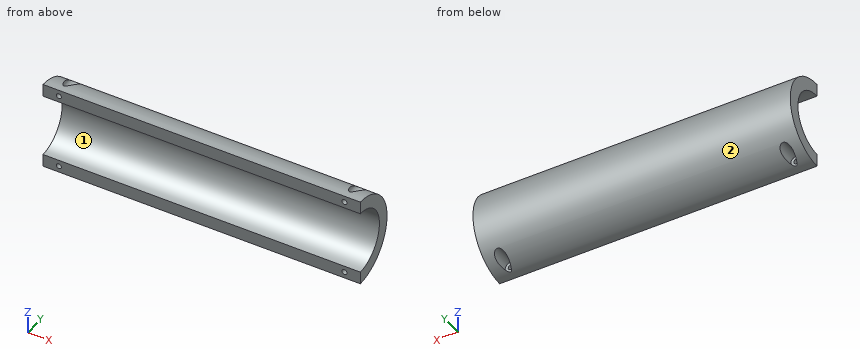
from build123d import *

# Parameters (mm, degrees)
AUFSATZ_LINEAR_AUSTRAGEN1_DEPTH = 200
SKIZZE2_R                       = 1.6
SCHNITT_LINEAR_AUSTRAGEN1_DEPTH = 204.882318998
SCHNITT_LINEAR_START            = -5
SKIZZE3_R                       = 3.5
SCHNITT_LINEAR_AUSTRAGEN2_DEPTH = 199.882319124


with BuildPart() as part:
    # Skizze1 → Aufsatz-Linear austragen1 (new body)
    with BuildSketch(Plane(origin=(0, 0, 0), x_dir=(0, 0, -1), z_dir=(1, 0, 0))):
        with BuildLine():
            Line((-28, 0), (-20, 0))
            ThreePointArc((-20, 0), (0, 20), (20, 0))
            Line((20, 0), (28, 0))
            ThreePointArc((28, 0), (0, 28), (-28, 0))
        make_face()
    extrude(amount=AUFSATZ_LINEAR_AUSTRAGEN1_DEPTH)

    # Skizze2 → Schnitt-Linear austragen1 (cut, through all)
    with BuildSketch(Plane.XZ):
        with Locations(Location((10, 24, 0), (0, 0, 270))):
            Circle(SKIZZE2_R)
        with Locations(Location((190, 24, 0), (0, 0, 270))):
            Circle(SKIZZE2_R)
        with Locations(Location((190, -24, 0), (0, 0, 270))):
            Circle(SKIZZE2_R)
        with Locations(Location((10, -24, 0), (0, 0, 270))):
            Circle(SKIZZE2_R)
    extrude(amount=-SCHNITT_LINEAR_AUSTRAGEN1_DEPTH, mode=Mode.SUBTRACT)

    # Skizze3 → Schnitt-Linear austragen2 (cut, through all)
    with BuildSketch(Plane.XZ.offset(SCHNITT_LINEAR_START)):
        with Locations(Location((10, 24, 0), (0, 0, 270))):
            Circle(SKIZZE3_R)
        with Locations(Location((190, 24, 0), (0, 0, 270))):
            Circle(SKIZZE3_R)
        with Locations(Location((190, -24, 0), (0, 0, 270))):
            Circle(SKIZZE3_R)
        with Locations(Location((10, -24, 0), (0, 0, 270))):
            Circle(SKIZZE3_R)
    extrude(amount=-SCHNITT_LINEAR_AUSTRAGEN2_DEPTH, mode=Mode.SUBTRACT)


solid = part.part
CAD build for the part. Positions are in the model's coordinates, mm. Face numbers are marked on the shaded views. Round coordinates to 2 decimals unless told otherwise and drop trailing zeros. Loops run counter-clockwise (first coordinate to the right, second up) from the corner with the lowest first, then second, coordinate; pieces in that order, holes last. Notation, with made-up numbers: M 72.5,-0.5 L 90.5,-0.5 A16 ccw 90.5,6.5 Z; hole C 47.5,72 d10. An arc over 180 degrees is marked long. One line per question, with ' | ' between items. Start each with the question number.
Item 1: Cut at D-D, the plane z = 0. Write the cut outline in (x, y).
Item 2: Cut at C-C, the plane x = 113.5. Write the cut outline in (y, z), plus the area to 3 significant figures.
Item 3: Wall check: line 1 (X direction, y = 3.6, z = 24); line 2 (X direction, y = 13.5, z = 24); line 3 (Z direction, x = 190, y = 1.75). Give the ranges that are in metal, low to high.
Item 4: Two-plate mould, pull along Z, no slides. Class the marked faces 1 and 2: pulls with the +Z half, pulls with the -Z half, needs draft (parallel to the pull), parting line crosses it, or undercut.
Item 5: Cut at B-B, the plane y = 14.5. Write the cut outline in (x, z), plus the area to 3 significant figures.
Item 6: Pin check, flat tips, straight feed: pin 1 Ø3 at (y, z) = (11.5, -20.5) entering from -X; pin 2 Ø11 at (x, z) = (10, -24) entering from +Y; pin 3 Ø12 at (y, z) = (6.5, -10) entering from -X; pin 4 Ø5.5 at (x, z) = (11, 22.5) entering from +Y. Stop position of each tip, or through.
Item 7: Cut at A-A, the plane y = 3. Write the cut outline in (x, z), plus the area to 3 significant figures.
Responses:
1) outline: M 0,20 L 200,20 L 200,28 L 0,28 Z
2) outline: M 0,-28 A28 ccw 0,28 L 0,20 A20 cw 0,-20 Z | area: 603 mm²
3) line 1: x = 0 to 8.4, 11.6 to 188.4, 191.6 to 200 | line 2: x = 0 to 6.5, 13.5 to 186.5, 193.5 to 200 | line 3: z = -27.95 to -25.6, -22.4 to -19.92, 19.92 to 22.4, 25.6 to 27.95
4) face 1: undercut | face 2: parting line crosses it
5) outline: M 0,-23.95 L 6.5,-23.95 A3.5 cw 13.5,-23.95 L 186.5,-23.95 A3.5 cw 193.5,-23.95 L 200,-23.95 L 200,-13.77 L 0,-13.77 Z; M 0,13.77 L 200,13.77 L 200,23.95 L 193.5,23.95 A3.5 cw 186.5,23.95 L 13.5,23.95 A3.5 cw 6.5,23.95 L 0,23.95 Z | area: 4,000 mm²
6) pin 1: stops at x = 0 | pin 2: stops at y = 21.02 | pin 3: passes through | pin 4: stops at y = 19.85
7) outline: M 0,-27.84 L 200,-27.84 L 200,-19.77 L 0,-19.77 Z; M 0,19.77 L 200,19.77 L 200,27.84 L 0,27.84 Z; hole C 10,-24 d3.2; hole C 10,24 d3.2; hole C 190,-24 d3.2; hole C 190,24 d3.2 | area: 3,190 mm²
